Autodesk Inventor part; units mm, degrees
ref_plane "YZ Plane" through (0, 0, 0) normal (1, 0, 0) x (0, 1, 0)
ref_plane "XZ Plane" through (0, 0, 0) normal (0, 1, 0) x (-1, 0, 0)
ref_plane "XY Plane" through (0, 0, 0) normal (0, 0, 1) x (1, 0, 0)
sketch "스케치1" plane through (0, 0, 0) normal (0, 0, 1) x (1, 0, 0)
  line L0 (-10, 0) -> (10, 0) construction
  line L1 (0, 0) -> (0, 20) construction
  line L2 (0, 20) -> (10, 0) construction
  line L3 (0, 20) -> (11.7082, 1.0557)
  line L4 (0, 20) -> (5.8657, 4.0994) construction
  line L5 (7.8647, -1.3197) -> (11.7082, 1.0557)
  line L6 (7.8647, -1.3197) -> (7.0141, -1.8454)
  line L7 (7.0141, -1.8454) -> (3.9324, -1.8454)
  line L8 (3.9324, -1.8454) -> (3.9324, -3.5)
  line L9 (3.9324, -3.5) -> (0, -3.5)
  line L10 (8.7322, 5.871) -> (4.8959, 3.5)
  line L11 (4.8959, 3.5) -> (0, 3.5)
  line L12 (0, 3.5) -> (0, -3.5)
  line L13 (5.8657, 4.0994) -> (7.8647, -1.3197)
  point P0 (5.8657, 4.0994)
  dimension "d0" = 20
  dimension "d1" = 20
  dimension "d4" = 2
  dimension "d5" = 2.5
  dimension "d6" = 1
  dimension "d8" = 3
  dimension "d11" = 3.5
  dimension "d12" = 7
  dimension "d40" = 4.5557
  dimension "d41" = 23.4164
revolve "회전1" add sketch "스케치1" angle 360 about axis through (0, 3.5, 0) along (0, -1, 0)
sketch "스케치4" plane through (0, 3.5, 0) normal (0, 1, 0) x (1, 0, 0)
  circle A0 centre (0, 0) radius 2.5
  dimension "d35" = 5
extrude "돌출1" cut sketch "스케치4" against normal blind 30.75
ref_plane "작업 평면4" through (7.8647, -1.3197, 0) normal (-0.5257, 0.8507, 0) x (-0.8507, -0.5257, 0)
sketch "스케치9" plane through (7.8647, -1.3197, 0) normal (-0.5257, 0.8507, 0) x (-0.8507, -0.5257, 0)
  ellipse E0 centre (5.4413, 0) end of major axis (5.4413, 11.7082) minor radius 9.9596 construction
  ellipse E1 centre (5.4413, 0) end of major axis (5.4413, 7.2082) minor radius 5.4596 (0.3405, 2.57) -> (0.0422, -1.07) ccw
  line L0 (-4.5183, 0) -> (-0.0183, 0)
  line L1 (-5.127, 1.07) -> (2.577, 1.07) construction
  line L2 (-5.5914, 1.57) -> (2.9534, 1.57) construction
  line L3 (-5.0964, 2.57) -> (1.9809, 2.57) construction
  arc A0 (-4.2754, 2.57) -> (0.0422, 1.07) centre (0.3783, 9.0013) ccw
  arc A1 (0.0422, -1.07) -> (-4.2754, -2.57) centre (0.3783, -9.0013) ccw
  line L4 (-4.2754, 2.57) -> (-6.6392, 2.57)
  line L5 (-6.6392, 2.57) -> (-6.6392, -2.57)
  line L6 (-6.6392, -2.57) -> (-4.2754, -2.57)
  point P0 (5.9964, 0)
  dimension "d55" = 1.57
  dimension "d56" = 4.5
  dimension "d57" = 0.5
  dimension "d58" = 1
properties part number "베벨기어 002"
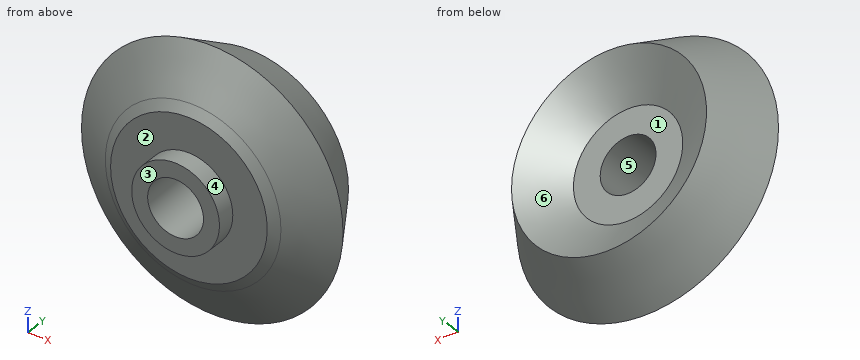
Model file for the job. Use its own axes, mm. Face numbers are marked on the shaded views. A direction names the side the tool comes from. Coordinates: 2 decimals unless noted, no trailing zeros. Write each loop counter-clockwise with the first axis right and the second up, starting at its lowest first coordinate (ties: lowest second). Pieces come first, ordered by that corner, then holes. Notation, with made-up numbers: (-11, 47) -> (40, 47) arc R14 ccw to (40, 63) -> close; hole circle Ø11 at (47.25, -16.5). An arc over 180 degrees is marked (long way). One line per item, written item: value. Start each with the question number.
1) Slice it at D-D on y = 5.25. Write the cut outline in (x, z), then the cut area to 3 significant figures.
2) Slice it at A-A on z = 0. Write the cut outline in (x, y).
3) Flat gauge pins, fed straight in: pin 1 Ø4 at (x, y) = (4.5, -0.5) entering from -Z; pin 2 Ø3 at (x, z) = (6.5, 1) entering from -Y; pin 3 Ø5 at (x, z) = (5, 6.5) entering from +Y; pin 4 Ø2 at (x, y) = (-6, 4) entering from +Z. Where does each tip first touch, or does it go through?
4) Slice it at C-C on y = 0. Write the cut outline in (x, z), then the cut area to 3 significant figures.
5) Slice it at B-B on x = 0. Write the cut outline in (y, z).
6) Probe probe 1 along X at (y, z) = (2.75, 2); probe 2 along X at (y, z) = (2, 0); probe 3 along Y at (x, z) = (-4.25, 0.5). List the from-to ranges inside material, lowest first.
7) Which spindle directions (+Z, -Z, +X, -X, +Y, -Y) get a long thin tool onto all of the face, cutting with end or side? Do the marked faces 1 and 2. Say none if no direction does.
8) Pull direction Z, two halves, no side cores. Call the marked faces 3, 4, 5 and 6: +Z half, -Z half, draft (parallel to the pull), parting line (faces both ways), or undercut.
Answers follow:
1. outline: circle Ø18.23 at (0, 0); hole circle Ø15.45 at (0, 0)
1. area: 73.5 mm2
2. outline: (-11.71, 1.06) -> (-7.86, -1.32) -> (-7.01, -1.85) -> (-3.93, -1.85) -> (-3.93, -3.5) -> (-2.5, -3.5) -> (-2.5, 3.5) -> (-4.9, 3.5) -> (-8.73, 5.87) -> close; (2.5, -3.5) -> (3.93, -3.5) -> (3.93, -1.85) -> (7.01, -1.85) -> (7.86, -1.32) -> (11.71, 1.06) -> (8.73, 5.87) -> (4.9, 3.5) -> (2.5, 3.5) -> close
3. pin 1: z = -11.25
3. pin 2: y = -1.85
3. pin 3: y = 5.87
3. pin 4: z = 8.87
4. outline: circle Ø20 at (0, 0); hole circle Ø5 at (0, 0)
4. area: 295 mm2
5. outline: (-3.5, -3.93) -> (-1.85, -3.93) -> (-1.85, -7.01) -> (-1.32, -7.86) -> (1.06, -11.71) -> (5.87, -8.73) -> (3.5, -4.9) -> (3.5, -2.5) -> (-3.5, -2.5) -> close; (-3.5, 2.5) -> (3.5, 2.5) -> (3.5, 4.9) -> (5.87, 8.73) -> (1.06, 11.71) -> (-1.32, 7.86) -> (-1.85, 7.01) -> (-1.85, 3.93) -> (-3.5, 3.93) -> close
6. probe 1: -10.47 to -1.5, 1.5 to 10.47
6. probe 2: -11.12 to -2.5, 2.5 to 11.12
6. probe 3: -1.85 to 3.5
7. face 1: +Y
7. face 2: -Y
8. face 3: draft
8. face 4: parting line
8. face 5: undercut
8. face 6: undercut
